```python
from build123d import *

# Parameters (mm, degrees)
BOSS_EXTRUDE1_DEPTH      = 115
CUT_EXTRUDE1_START       = -15
CUT_EXTRUDE1_DEPTH       = 15
CUT_EXTRUDE2_DEPTH       = 58
SKETCH6_W                = 33
SKETCH6_H                = 40
CUT_EXTRUDE3_DEPTH       = 58
BOSS_EXTRUDE2_DEPTH      = 5
BOSS_EXTRUDE2_DEPTH_BACK = 15
SKETCH7_W                = 47
SKETCH7_H                = 15
BOSS_EXTRUDE3_DEPTH      = 5
BOSS_EXTRUDE3_DEPTH_BACK = 15
SKETCH8_W                = 47
SKETCH8_H                = 15


with BuildPart() as part:
    # Sketch2 → Boss-Extrude1 (new body)
    with BuildSketch(Plane.XY):
        with BuildLine():
            Line((-20, -51.23475383), (-20, -26.916730868))
            Line((-20, -26.916730868), (20, -26.916730868))
            Line((20, -26.916730868), (20, -11.916730868))
            Line((20, -11.916730868), (0, -11.916730868))
            ThreePointArc((0, -11.916730868), (-7.071067812, -8.98779868), (-10, -1.916730868))
            Line((-10, -1.916730868), (-10, 54.083269132))
            ThreePointArc((-10, 54.083269132), (-54.753734942, 5.198895061), (-20, -51.23475383))
        make_face()
    extrude(amount=BOSS_EXTRUDE1_DEPTH)

    # Sketch3 → Cut-Extrude1 (cut)
    with BuildSketch(Plane.XY.offset(115).offset(CUT_EXTRUDE1_START)):
        with BuildLine():
            Line((-54.666698166, -6.045834235), (20, -21.916730868))
            Line((20, -21.916730868), (20, -11.916730868))
            Line((20, -11.916730868), (0, -11.916730868))
            ThreePointArc((0, -11.916730868), (-7.071067812, -8.98779868), (-10, -1.916730868))
            Line((-10, -1.916730868), (-10, 54.083269132))
            ThreePointArc((-10, 54.083269132), (-44.151135103, 32.797519253), (-54.666698166, -6.045834235))
        make_face()
    extrude(amount=CUT_EXTRUDE1_DEPTH, mode=Mode.SUBTRACT)

    # Sketch4 → Cut-Extrude2 (cut)
    with BuildSketch(Plane(origin=(0, -11.916730868, 0), x_dir=(1, 0, 0), z_dir=(0, 1, 0))):
        with BuildLine():
            Line((15, -10), (15, -90))
            ThreePointArc((15, -90), (10, -95), (5, -90))
            Line((5, -90), (5, -10))
            ThreePointArc((5, -10), (10, -5), (15, -10))
        make_face()
    extrude(amount=-CUT_EXTRUDE2_DEPTH, mode=Mode.SUBTRACT)

    # Sketch6 → Cut-Extrude3 (cut)
    with BuildSketch(Plane(origin=(-10, 0, 0), x_dir=(0, 0, -1), z_dir=(1, 0, 0))):
        with Locations((-53.5, 34.083269132)):
            Rectangle(SKETCH6_W, SKETCH6_H)
    extrude(amount=-CUT_EXTRUDE3_DEPTH, mode=Mode.SUBTRACT)

    # Sketch7 → Boss-Extrude2 (add, two sides: drawn at the far end of the back side and taken through both)
    with BuildSketch(Plane(origin=(-10, 0, 0), x_dir=(0, 0, -1), z_dir=(1, 0, 0)).offset(-BOSS_EXTRUDE2_DEPTH_BACK)):
        with Locations((-13.5, 31.583269132)):
            Rectangle(SKETCH7_W, SKETCH7_H)
    extrude(amount=BOSS_EXTRUDE2_DEPTH + BOSS_EXTRUDE2_DEPTH_BACK)

    # Sketch8 → Boss-Extrude3 (add, two sides: drawn at the far end of the back side and taken through both)
    with BuildSketch(Plane(origin=(-10, 0, 0), x_dir=(0, 0, -1), z_dir=(1, 0, 0)).offset(-BOSS_EXTRUDE3_DEPTH_BACK)):
        with Locations((-93.5, 31.583269132)):
            Rectangle(SKETCH8_W, SKETCH8_H)
    extrude(amount=BOSS_EXTRUDE3_DEPTH + BOSS_EXTRUDE3_DEPTH_BACK)


solid = part.part
```
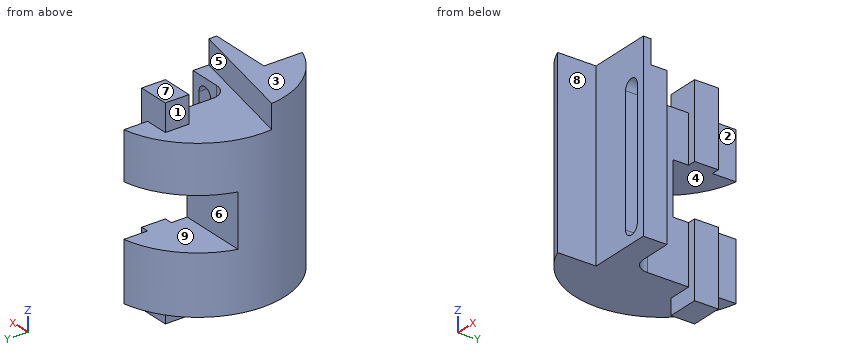
For this review, take the finished solid that the model builds, in its own axes (mm). Face numbers are marked on the shaded views. A direction names the side the tool comes from. Give positions to 0.01 mm unless a question says otherwise; leave off trailing zeros. Write each loop counter-clockwise with the first axis right and the second up, starting at its lowest first coordinate (ties: lowest second). Pieces come first, ordered by that corner, then holes. Notation, with made-up numbers: M -31.75,-19.5 L -22.75,-19.5 A26 cw -22.75,3.5 Z; hole C -34,10 d1. An arc over 180 degrees is marked long. Answer as a JSON object with one key per item and string values. Group by question number.
Item 1: Consider section C-C on z = 97.5. Write out the cut boundary in (x, y), plus the area to 3 significant figures.
Item 2: Consider section D-D on y = 17.5. Write out the cut boundary in (x, z), plus the area to 3 significant figures.
Item 3: Tool access review of the marked faces 1, 2, 3, 4 and 5: name each direction out of +Z, -Z, +X, -X, +Y, -Y from which nothing blocks a thin tool from reaching the whole face with its end or side.
Item 4: Consider section A-A on z = 22.5. Write out the cut boundary in (x, y).
Item 5: For probe 1 along Z at (x, y) = (-9, 31); probe 2 along Z at (x, y) = (-11, 10.5); probe 3 along Z at (x, y) = (-41, -34), list the stretches that pass through material, from the lowest coordinate up. Write a range as [from, to].
Item 6: For pin 1 Ø8 at (y, z) = (29.5, -5.5) entering from -X; pin 2 Ø10 at (y, z) = (3.5, 14.5) entering from +X; pin 3 Ø16.5 at (y, z) = (44, 82.5) entering from +X, all flat-tipped, find the tip position at first contact; note any pin that passes through.
Item 7: Draft analysis for pull direction Z (two halves, no side actions). For the marked faces 6, 7, 8 and 9, state which applies: +Z half, -Z half, draft (parallel to the pull), parting line (faces both ways), or undercut.
Item 8: Consider section B-B on x = 10. Write out the cut boundary in (y, z), plus the area to 3 significant figures.
Check result:
{
 "1": {"outline": "M -20,-51.23 L -20,-26.92 L 20,-26.92 L 20,-11.92 L 0,-11.92 A10 cw -10,-1.92 L -10,24.08 L -5,24.08 L -5,39.08 L -10,39.08 L -10,54.08 A55 ccw Z", "area": "3,950 mm^2"},
 "2": {"outline": "M -52.14,0 L -10,0 L -10,37 L -52.14,37 Z; M -52.14,70 L -10,70 L -10,100 L -52.14,100 Z", "area": "2,820 mm^2"},
 "3": {"face 1": "+Z, -X, +Y", "face 2": "+Z, -Z, +X, +Y", "face 3": "+Z, +X, -X, -Y", "face 4": "+X, -X, +Y", "face 5": "+Z, +X"},
 "4": {"outline": "M -20,-51.23 L -20,-26.92 L 5,-26.92 L 5,-11.92 L 0,-11.92 A10 cw -10,-1.92 L -10,24.08 L -5,24.08 L -5,39.08 L -10,39.08 L -10,54.08 A55 ccw Z; M 15,-26.92 L 20,-26.92 L 20,-11.92 L 15,-11.92 Z"},
 "5": {"probe 1": "z = [-10, 37], [70, 117]", "probe 2": "z = [0, 100]", "probe 3": "z = [0, 115]"},
 "6": {"pin 1": "stops at x = -25", "pin 2": "stops at x = -10", "pin 3": "stops at x = -5"},
 "7": {"face 6": "undercut", "face 7": "+Z half", "face 8": "draft", "face 9": "undercut"},
 "8": {"outline": "M -26.92,0 L -11.92,0 L -11.92,5 L -26.92,5 Z; M -26.92,95 L -11.92,95 L -11.92,100 L -19.79,100 L -19.79,115 L -26.92,115 Z", "area": "257 mm^2"}
}
